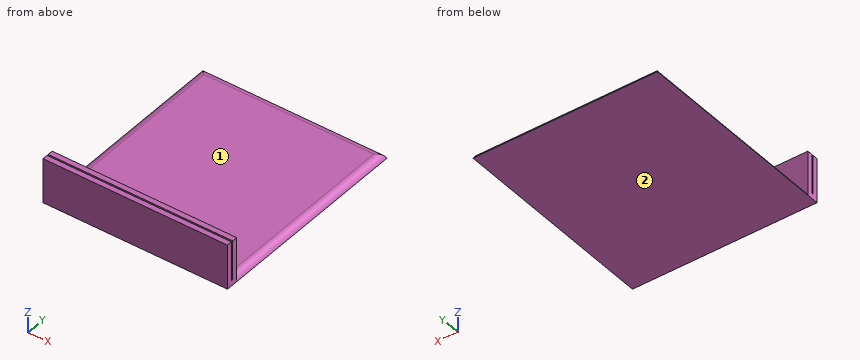
from build123d import *

# Parameters (mm, degrees)
F0_W        = 1.9147001281
F0_H        = 2
F0_W_2      = 0.6
F0_W_3      = 2
F0_H_2      = 15
F0_W_4      = 75.4852998719
F1_DEPTH    = 35
F2_T1_DEPTH = 82.5563676837
F2_T3_DEPTH = 84.1421356237


# Not quite as in the source:
# - a fillet or chamfer that OpenCascade refuses, or shapes differently, is made with other operations: its cross-section is extruded or revolved along the edge and cut away or added


with BuildPart() as f1:
    # F0 (on Right) → F1 (new body, symmetric)
    with BuildSketch(Plane.YZ):
        Polygon((-48.8228555396, -4.8070274784), (-48.8228555396, -2.8070274784), (-46.9081554115, -2.8070274784), (-46.9081554115, 12.1929725216), (-48.9081554115, 12.1929725216), (-48.9081554115, -4.8070274784), align=None)
        with Locations((-47.8655054756, -3.8070274784)):
            Rectangle(F0_W, F0_H)
        with Locations((-46.6081554115, -3.8070274784)):
            Rectangle(F0_W_2, F0_H)
        with Locations((-45.3081554115, 4.6929725216)):
            Rectangle(F0_W_3, F0_H_2)
        with Locations((-45.3081554115, -3.8070274784)):
            Rectangle(F0_W_3, F0_H)
        with Locations((-6.5655054756, -3.8070274784)):
            Rectangle(F0_W_4, F0_H)
    extrude(amount=F1_DEPTH, both=True)

    # F2: fillet of radius 3 on 3 edges, made by hand

    # F2_s2 → F2_t1 (cut)
    with BuildSketch(Plane.XZ.offset(-38.2482122722)):
        with BuildLine():
            ThreePointArc((32.1715728753, -2.8070274784), (33.9036236828, -3.3575377356), (35, -4.8070274784))
            Line((35, -4.8070274784), (35, -2.8070274784))
            Line((35, -2.8070274784), (32.1715728753, -2.8070274784))
        make_face()
        with BuildLine():
            ThreePointArc((-32.1715728753, -2.8070274784), (-33.9036236828, -3.3575377356), (-35, -4.8070274784))
            Line((-35, -4.8070274784), (-35, -2.8070274784))
            Line((-35, -2.8070274784), (-32.1715728753, -2.8070274784))
        make_face()
    extrude(amount=F2_T1_DEPTH, mode=Mode.SUBTRACT)

    # F2_s4 → F2_t3 (cut)
    with BuildSketch(Plane.YZ.offset(-42.0710678119)):
        with BuildLine():
            ThreePointArc((28.3487173356, -2.8070274784), (30.0807681432, -3.3575377356), (31.1771444604, -4.8070274784))
            Line((31.1771444604, -4.8070274784), (31.1771444604, -2.8070274784))
            Line((31.1771444604, -2.8070274784), (28.3487173356, -2.8070274784))
        make_face()
    extrude(amount=F2_T3_DEPTH, mode=Mode.SUBTRACT)


solid = f1.part
Work out the finished part from the listing and answer in its coordinate system (mm). Face numbers are marked on the shaded views. A direction names the side the tool comes from. Round coordinates to 2 decimals unless told otherwise and drop trailing zeros. Write each loop counter-clockwise with the first axis right and the second up, starting at its lowest first coordinate (ties: lowest second). Pieces come first, ordered by that corner, then holes. Notation, with made-up numbers: (43, -35.5) -> (69, -35.5) arc R32 ccw to (69, -4.5) -> close; hole circle Ø8 at (74.5, 10). An arc over 180 degrees is marked (long way). Write each question's results on one line, items separated by ' | '.
Item 1: Flat-ended cylindrical pins translate along their axes: P1, Ø8.5, axis at x = -12, z = 7.5, coming from the +Y side; P2, Ø1, axis at x = -25, y = 18.5, coming from the +Z side. Find the tip coordinate at first contact, or state that the pin passes through.
Result set:
P1: y = -44.31 | P2: z = -2.81
Item 2: Which of the six approach directions +Z, -Z, +X, -X, +Y, -Y give full straight-line access (tool end or side, diameter ignored) to the marked faces 1 and 2?
Result set:
face 1: +Z, +X, -X, +Y | face 2: -Z, +X, -X, +Y, -Y
Item 3: A cutting plane is placed at B-B, the plane x = 0. Determine the outline of the cut face in (y, z), plus the area to 3 significant figures.
Result set:
outline: (-48.91, -4.81) -> (31.18, -4.81) arc R3 ccw to (28.35, -2.81) -> (-44.31, -2.81) -> (-44.31, 12.19) -> (-46.31, 12.19) -> (-46.31, -2.81) -> (-46.91, -2.81) -> (-46.91, 12.19) -> (-48.91, 12.19) -> close | area: 219 mm^2
Item 4: A cutting plane is placed at A-A, the plane z = 9.5. Determine the outline of the cut face in (x, y), plus the area to 3 significant figures.
Result set:
outline: (-35, -48.91) -> (35, -48.91) -> (35, -46.91) -> (-35, -46.91) -> close; (-35, -46.31) -> (35, -46.31) -> (35, -44.31) -> (-35, -44.31) -> close | area: 280 mm^2
Item 5: A cutting plane is placed at C-C, the plane y = -3. Determine the outline of the cut face in (x, z).
Result set:
outline: (-35, -4.81) -> (35, -4.81) arc R3 ccw to (32.17, -2.81) -> (-32.17, -2.81) arc R3 ccw to start
Item 6: Find the intervals of material crossed by line 1 along Y through (x, z) = (3.5, 10.25); line 2 along Z through (x, y) = (-7.5, 3); line 3 along X through (y, z) = (-37.5, -3.5), in increasing order. Write a range as [from, to].
Result set:
line 1: [-48.91, -46.91], [-46.31, -44.31] | line 2: [-4.81, -2.81] | line 3: [-34.09, 34.09]
